Print and shaded views of the part. All mm, measured from the part's lowest x, y and z. Give positions to 0.01 mm unless a question says otherwise; leave off trailing zeros. Write each loop counter-clockwise with the first axis right and the second up, starting at its lowest first coordinate (ties: lowest second). Pieces come first, ordered by that corner, then holes. Notation, with made-up numbers: (38, 57) - (54, 57) arc R22 ccw to (54, 66) - close; hole circle Ø2 at (-22, 46). An arc over 180 degrees is marked (long way). Use one line per item in the form item = value. Start each with the question number.
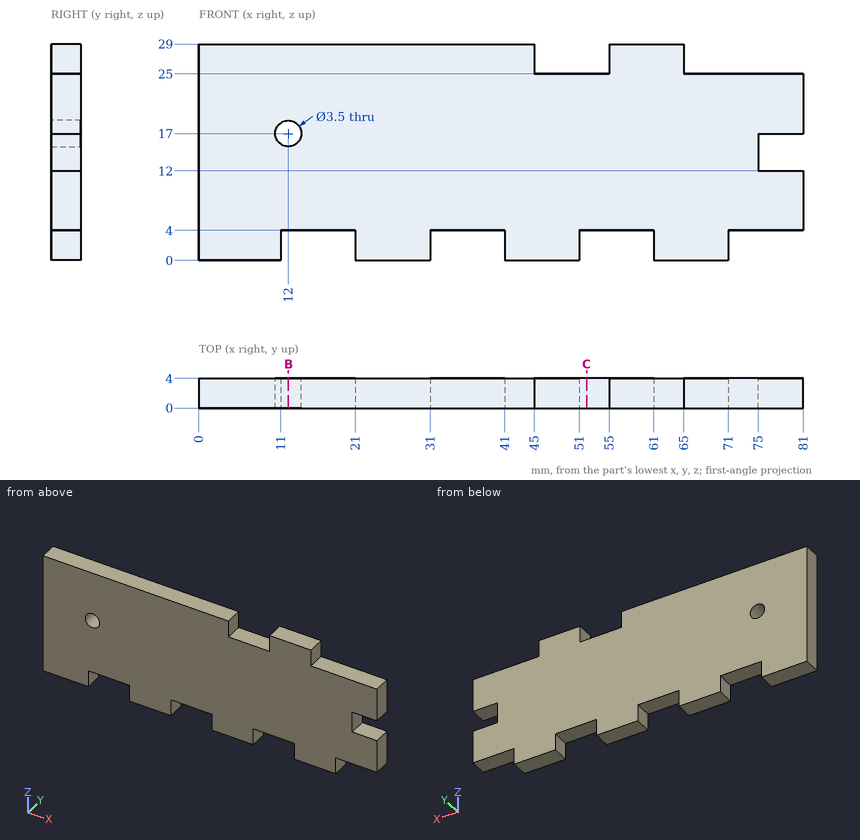
(1) Wall check: line 1 (X direction, y = 0.4, z = 2); line 2 (Z direction, x = 71.5, y = 1.95); line 3 (Z direction, x = 10.5, y = 1.35). Give the ranges that are in metal, low to high. Write a range as from..to.
(2) Pin check, flat tips, straight feed: pin 1 Ø1.2 at (x, y) = (55.5, 2.5) entering from -Z; pin 2 Ø1.2 at (x, y) = (52.5, 2) entering from +Z; pin 3 Ø1.2 at (y, z) = (2.5, 2) entering from +X. Stop position of each tip, or through.
(3) Cut at B-B, the plane x = 12. Give the cut face in (y, z), then the cut area to 3 significant figures.
(4) Cut at C-C, the plane x = 52. Give the cut face in (y, z), then the cut area to 3 significant figures.
Solution:
q1.line_1 = 0..11, 21..31, 41..51, 61..71
q1.line_2 = 4..25
q1.line_3 = 0..16.1, 17.9..29
q2.pin_1 = 4
q2.pin_2 = 25
q2.pin_3 = 71
q3.outline = (0, 4) - (4, 4) - (4, 15.25) - (0, 15.25) - close; (0, 18.75) - (4, 18.75) - (4, 29) - (0, 29) - close
q3.area = 86.0 mm2
q4.outline = (0, 4) - (4, 4) - (4, 25) - (0, 25) - close
q4.area = 84.0 mm2
